Autodesk Inventor part; units mm, degrees
ref_plane "YZ Plane" through (0, 0, 0) normal (1, 0, 0) x (0, 1, 0)
ref_plane "XZ Plane" through (0, 0, 0) normal (0, 1, 0) x (-1, 0, 0)
ref_plane "XY Plane" through (0, 0, 0) normal (0, 0, 1) x (1, 0, 0)
sketch "Skizze1" plane through (0, 0, 0) normal (0, 0, 1) x (1, 0, 0)
  circle A0 centre (16.76, 0) radius 1.25
  circle A1 centre (-16.76, 0) radius 1.25
  line L0 (-6.25, 16) -> (-11.9414, 16)
  line L1 (-2.25, 20) -> (-6.25, 16)
  line L2 (2.25, 20) -> (-2.25, 20)
  line L3 (6.25, 16) -> (2.25, 20)
  line L4 (11.9414, 16) -> (6.25, 16)
  line L5 (11.9414, 16) -> (12.9414, 15)
  line L6 (12.9414, -15) -> (12.9414, 15)
  line L7 (11.9414, -16) -> (12.9414, -15)
  line L8 (-11.9414, -16) -> (11.9414, -16)
  line L9 (-11.9414, -16) -> (-12.9414, -15)
  line L10 (-12.9414, 15) -> (-12.9414, -15)
  line L11 (-12.9414, 15) -> (-11.9414, 16)
  circle A2 centre (0, 0) radius 20.5786
  point P0 (0, 0)
extrude "Extrusion1" add sketch "Skizze1" along normal blind 4 contours L1 L2 L3 L4 L5 L6 L7 L8 L9 L10 L11 L0 | A2
sketch "Skizze2" plane through (0, 0, 4) normal (0, 0, 1) x (1, 0, 0)
  point P0 (0, 0)
sketch "Skizze3" plane through (0, 0, 4) normal (0, 0, 1) x (1, 0, 0)
  line L0 (-12.1, -11.9394) -> (-9.9, -11.9394)
  line L1 (-9.9, -11.9394) -> (-9.9, 11.9394)
  line L2 (-9.9, 11.9394) -> (-12.1, 11.9394)
  line L3 (-12.1, 11.9394) -> (-12.1, -11.9394)
  line L4 (-7.7, 14.502) -> (-5.5, 14.502)
  line L5 (-5.5, 14.502) -> (-5.5, -14.502)
  line L6 (-5.5, -14.502) -> (-7.7, -14.502)
  line L7 (-7.7, -14.502) -> (-7.7, 14.502)
  line L8 (-3.3, 15.4709) -> (-1.1, 15.4709)
  line L9 (-1.1, 15.4709) -> (-1.1, -15.4709)
  line L10 (-1.1, -15.4709) -> (-3.3, -15.4709)
  line L11 (-3.3, -15.4709) -> (-3.3, 15.4709)
  circle A0 centre (-16.76, 0) radius 1.25
  circle A1 centre (16.76, 0) radius 1.25
  circle A2 centre (0, 0) radius 20.5786
  line L12 (-16.76, 0) -> (0, 0) construction
  circle A3 centre (0, 0) radius 15.51 construction
  line L13 (0, 0) -> (0, 15.51)
  point P0 (0, 0)
  dimension "d2" = 2.2
  dimension "d3" = 2.2
  dimension "d4" = 2.2
  dimension "d5" = 2.2
  dimension "d6" = 2.2
  dimension "d7" = 1.1
ref_plane "Arbeitsebene1" through (0, 0, 4) normal (1, 0, 0) x (0, 1, 0)
extrude "Extrusion2" cut sketch "Skizze3" against normal through all contours L3 L2 L1 L0 | L4 L5 L6 L7 | L8 L9 L10 L11
mirror "Spiegeln1" about plane through (0, 0, 4) normal (1, 0, 0) of "Extrusion2"
sketch "Skizze4" plane through (0, 0, 4) normal (0, 0, 1) x (1, 0, 0)
  line L0 (5.5, -14.502) -> (5.5, 14.502)
  line L1 (5.5, 14.502) -> (7.7, 14.502)
  line L2 (7.7, 14.502) -> (7.7, -14.502)
  line L3 (7.7, -14.502) -> (5.5, -14.502)
  line L4 (1.1, -15.4709) -> (1.1, 15.4709)
  line L5 (1.1, 15.4709) -> (3.3, 15.4709)
  line L6 (3.3, 15.4709) -> (3.3, -15.4709)
  line L7 (3.3, -15.4709) -> (1.1, -15.4709)
  line L8 (9.9, 11.9394) -> (12.1, 11.9394)
  line L9 (12.1, 11.9394) -> (12.1, -11.9394)
  line L10 (12.1, -11.9394) -> (9.9, -11.9394)
  line L11 (9.9, -11.9394) -> (9.9, 11.9394)
  line L12 (-7.7, -14.502) -> (-7.7, 14.502)
  line L13 (-7.7, 14.502) -> (-5.5, 14.502)
  line L14 (-5.5, 14.502) -> (-5.5, -14.502)
  line L15 (-5.5, -14.502) -> (-7.7, -14.502)
  line L16 (-9.9, 11.9394) -> (-9.9, -11.9394)
  line L17 (-9.9, -11.9394) -> (-12.1, -11.9394)
  line L18 (-12.1, -11.9394) -> (-12.1, 11.9394)
  line L19 (-12.1, 11.9394) -> (-9.9, 11.9394)
  line L20 (-3.3, -15.4709) -> (-3.3, 15.4709)
  line L21 (-3.3, 15.4709) -> (-1.1, 15.4709)
  line L22 (-1.1, 15.4709) -> (-1.1, -15.4709)
  line L23 (-1.1, -15.4709) -> (-3.3, -15.4709)
  circle A0 centre (-16.76, 0) radius 1.25
  circle A1 centre (16.76, 0) radius 1.25
  circle A2 centre (0, 0) radius 20.5786
  point P0 (0, 0)
hole "Bohrung1" at (-16.76, 0, 4) at (16.76, 0, 4) direction (0, 0, -1) diameter 3.2 end through all
sketch "Skizze5" plane through (0, 0, 4) normal (0, 0, 1) x (1, 0, 0)
  circle A0 centre (-16.76, 0) radius 1.6
  circle A1 centre (16.76, 0) radius 1.6
  line L0 (5.5, -14.502) -> (5.5, 14.502)
  line L1 (5.5, 14.502) -> (7.7, 14.502)
  line L2 (7.7, 14.502) -> (7.7, -14.502)
  line L3 (7.7, -14.502) -> (5.5, -14.502)
  line L4 (1.1, -15.4709) -> (1.1, 15.4709)
  line L5 (1.1, 15.4709) -> (3.3, 15.4709)
  line L6 (3.3, 15.4709) -> (3.3, -15.4709)
  line L7 (3.3, -15.4709) -> (1.1, -15.4709)
  line L8 (9.9, 11.9394) -> (12.1, 11.9394)
  line L9 (12.1, 11.9394) -> (12.1, -11.9394)
  line L10 (12.1, -11.9394) -> (9.9, -11.9394)
  line L11 (9.9, -11.9394) -> (9.9, 11.9394)
  line L12 (-7.7, -14.502) -> (-7.7, 14.502)
  line L13 (-7.7, 14.502) -> (-5.5, 14.502)
  line L14 (-5.5, 14.502) -> (-5.5, -14.502)
  line L15 (-5.5, -14.502) -> (-7.7, -14.502)
  line L16 (-9.9, 11.9394) -> (-9.9, -11.9394)
  line L17 (-9.9, -11.9394) -> (-12.1, -11.9394)
  line L18 (-12.1, -11.9394) -> (-12.1, 11.9394)
  line L19 (-12.1, 11.9394) -> (-9.9, 11.9394)
  line L20 (-3.3, -15.4709) -> (-3.3, 15.4709)
  line L21 (-3.3, 15.4709) -> (-1.1, 15.4709)
  line L22 (-1.1, 15.4709) -> (-1.1, -15.4709)
  line L23 (-1.1, -15.4709) -> (-3.3, -15.4709)
  circle A2 centre (0, 0) radius 20.5786
  point P0 (0, 0)
extrude "Extrusion3" add sketch "Skizze5" against normal up to surface (4 mm away) contours L0 L1 L2 L3 | L4 L5 L6 L7 | L8 L9 L10 L11 | L12 L13 L14 L15 | L16 L17 L18 L19 | L20 L21 L22 L23
sketch "Skizze6" plane through (0, 0, 4) normal (0, 0, 1) x (1, 0, 0)
  circle A0 centre (0, 0) radius 9
  circle A1 centre (0, 0) radius 7
  dimension "d20" = 18
  dimension "d21" = 2
extrude "Extrusion4" add sketch "Skizze6" along normal blind 10
sketch "Skizze9" plane through (0, 0, 4) normal (0, 0, 1) x (1, 0, 0)
  circle A0 centre (0, 0) radius 7
extrude "Extrusion6" cut sketch "Skizze9" against normal through all
sketch "Skizze10" plane through (0, 0, 14) normal (0, 0, 1) x (1, 0, 0)
  circle A0 centre (0, 0) radius 7
  circle A1 centre (0, 0) radius 9
  circle A2 centre (0, 0) radius 5
  dimension "d28" = 10
extrude "Extrusion7" add sketch "Skizze10" against normal blind 4 contours A0
chamfer "Fase1" distance 2 angle 45 1 edges at (-7, 0, 10)
fillet "Rundung1" radius 6 1 edges at (-9, 0, 4)
sketch "Skizze11" plane through (0, 0, 0) normal (0, 0, -1) x (-1, 0, 0)
  point P0 (0, 0)
chamfer "Fase2" distance 7 angle 45 1 edges at (-7, 0, 0)
fillet "Rundung2" radius 2 1 edges at (-20.5786, 0, 4)
sketch "Skizze7" plane through (0, 0, 14) normal (0, 0, 1) x (1, 0, 0)
  circle A0 centre (0, 0) radius 7
equation "\"d3\" = d2"
equation "\"d4\" = d3"
equation "\"d5\" = d4"
equation "\"d6\" = d3"
equation "\"d7\" = 0.5 * d2"
properties part number "Wrist_Cover_2" material "ABS-Kunststoff"
Work out the finished part from the listing and answer in its coordinate system (mm). A direction names the side the tool comes from. Round coordinates to 2 decimals unless told otherwise and drop trailing zeros.
1) A cutting plane is placed at A-A (y = 0). Give the number of separate pieces and of enclosed holes in the cut face, plus the area to 3 significant figures.
2) Straight lines are drawn through the part: line 1 (Y direction, x = 0, z = 11.65); line 2 (Z direction, x = 9, y = 15.5); line 3 (Y direction, x = 9, z = 1.5). For each, find the intervals that lie inside material, in ascending order.
3) The mould has two halves that part along Y. Classify faces 1 (the cylindrical face through (6.466, 2.681, 7.493)), 2 (the flat face through (-4.9, -13.4, 0)), 3 (the cylindrical face through (-1.172, -8.923, 11.972)): pulls with the +Y half, pulls with the -Y half, needs draft (parallel to the pull), parting line crosses it, or undercut.
4) A tool of negligible diameter and unlimited length cuts with its end or side. For faces 4 (the flat face through (-1.5, -15.1, 4)), 5 (the cylindrical face through (-15.167, -13.908, 0.986)), from which of +Z, -Z, +X, -X, +Y, -Y can it reach the whole face along a straight path? Write none if from no direction.
5) Given pin 1 Ø3 at (x, z) = (-11, 11) entering from -Y; pin 2 Ø12.5 at (x, y) = (0, 0) entering from -Z; pin 3 Ø13 at (x, y) = (0, 0) entering from -Z; pin 4 Ø6 at (x, z) = (-7.5, 8) entering from +Y, each flat-ended and moving along its own axis, determine where each tip first touches the part or whether it passes through.
Completed:
1. separate pieces: 4
1. enclosed holes: 0
1. area: 108 mm2
2. line 1: y = -9 to -5, 5 to 9
2. line 2: z = 0 to 4
2. line 3: y = -18.51 to -8.67, 8.67 to 18.51
3. face 1: undercut
3. face 2: needs draft
3. face 3: parting line crosses it
4. face 4: +Z
4. face 5: +Z, -Z
5. pin 1: passes through
5. pin 2: stops at z = 8.75
5. pin 3: stops at z = 8.5
5. pin 4: stops at y = 9.42
